from build123d import *

# Parameters (mm, degrees)
BOSS_EXTRUDE1_DEPTH = 25.9334
FILLET1_R           = 1.5748
CHAMFER1_SIZE       = 0.254
CHAMFER2_SIZE       = 0.254


with BuildPart() as part:
    # Sketch1 → Boss-Extrude1 (new body)
    with BuildSketch(Plane.XY):
        Polygon((0, 18.330871047), (-15.875, 9.165435523), (-15.875, -9.165435523), (0, -18.330871047), (15.875, -9.165435523), (15.875, 9.165435523), align=None)
    extrude(amount=BOSS_EXTRUDE1_DEPTH)

    # Sketch2 → Cut-Revolve1 (revolve, cut)
    with BuildSketch(Plane(origin=(0, 0, 0), x_dir=(0, 0, -1), z_dir=(1, 0, 0))):
        Polygon((-25.9334, 20.786742094), (-25.9334, 15.875), (-22.225, 15.875), (-21.566951336, 18.330871047), (-3.833048664, 18.330871047), (-3.175, 15.875), (0, 15.875), (0, 20.786742094), align=None)
        with BuildLine():
            Line((-25.9334, 10.5918), (-25.9334, 0))
            Line((-25.9334, 0), (0, 0))
            Line((0, 0), (0, 12.720416378))
            Line((0, 12.720416378), (-21.7932, 12.720416378))
            ThreePointArc((-21.7932, 12.720416378), (-21.972805122, 12.6460215), (-22.0472, 12.466416378))
            Line((-22.0472, 12.466416378), (-22.0472, 10.5918))
            Line((-22.0472, 10.5918), (-25.9334, 10.5918))
        make_face()
    revolve(axis=Axis((0, 0, 0), (0, 0, 1)), mode=Mode.SUBTRACT)

    # Fillet1
    fillet1_edges = [part.edges().sort_by_distance(p)[0] for p in [
        (0, -15.875, 25.9334),
    ]]
    fillet(fillet1_edges, radius=FILLET1_R)

    # Chamfer1
    chamfer1_edges = [part.edges().sort_by_distance(p)[0] for p in [
        (0, -15.875, 0),
    ]]
    chamfer(chamfer1_edges, length=CHAMFER1_SIZE)

    # Chamfer2
    chamfer2_edges = [part.edges().sort_by_distance(p)[0] for p in [
        (0, -10.5918, 25.9334),
        (0, -10.5918, 22.0472),
    ]]
    chamfer(chamfer2_edges, length=CHAMFER2_SIZE)


solid = part.part
Input: part model. Units: mm. Frame: model coordinates. A direction names the side the tool comes from. Give positions to 0.01 mm unless a question says otherwise; leave off trailing zeros. Order: outer loops, then holes, each group sorted by start corner. A loop starts at its lowest first (then second) coordinate and runs counter-clockwise, first axis right, second up. Notation, with made-up numbers: (6.5, 40) -> (16.5, 40) arc R18 cw to (16.5, 54) -> close; hole circle Ø1 at (-2, -39). An arc over 180 degrees is marked (long way). Use one line per item in the form item = value.
1) Reachability of faces 1 (the conical face through (14.235, -8.265, 3.332)), 2 (the cylindrical face through (4.87, 11.75, 11.05)) from +Z, -Z, +X, -X, +Y, -Y: full face, straight path, thin tool, end or side. Return the list, or none.
Response values:
face_1 = -Z, +X, -Y
face_2 = -Z
2) First-contact query: pin 1 Ø5 at (x, z) = (-3, 5.5) entering from +Y; pin 2 Ø6 at (y, z) = (-14, 21) entering from +X. Flat tips, straight axial feed; report the tip coordinate or a pass-through.
Response values:
pin_1 = 18.04
pin_2 = 12.7
3) Section A-A, the plane z = 21. Return loops of the section in (x, y) (3 decimals), and give its area (3 significant figures).
Response values:
outline = (-15.875, -9.165) -> (0, -18.331) -> (15.875, -9.165) -> (15.875, 9.165) -> (0, 18.331) -> (-15.875, 9.165) -> close; hole circle Ø25.441 at (0, 0)
area = 365 mm^2
4) Line query: probe 1 along X at (y, z) = (0, 24.25) (3 decimals); probe 2 along X at (y, z) = (-9.5, 12.5). Output: solid intervals per line, ascending.
Response values:
probe_1 = -15.875 to -10.592, 10.592 to 15.875
probe_2 = -15.3 to -8.46, 8.46 to 15.3
